Read the model definition and answer for the solid it produces. Units are mm, in the model's axes. A direction names the side the tool comes from. Round coordinates to 2 decimals unless told otherwise and drop trailing zeros. Write each loop counter-clockwise with the first axis right and the second up, starting at its lowest first coordinate (ties: lowest second). Pieces come first, ordered by that corner, then holes.
from build123d import *

# Parameters (mm, degrees)
SKETCH3_R           = 18.499963
BOSS_EXTRUDE1_DEPTH = 57.8000114
SKETCH4_R           = 2.999994
BOSS_EXTRUDE2_DEPTH = 20.00001334
SKETCH6_R           = 6.0000007
BOSS_EXTRUDE3_DEPTH = 5.0000154
SKETCH8_R           = 1.25000004
CUT_EXTRUDE3_DEPTH  = 8.89
SKETCH7_W           = 3.305573972
SKETCH7_H           = 0.499999
CUT_EXTRUDE4_DEPTH  = 13.9999974


with BuildPart() as part:
    # Sketch3 → Boss-Extrude1 (new body)
    with BuildSketch(Plane.XY):
        Circle(SKETCH3_R)
    extrude(amount=-BOSS_EXTRUDE1_DEPTH)

    # Sketch4 → Boss-Extrude2 (add)
    with BuildSketch(Plane.XY):
        Circle(SKETCH4_R)
    extrude(amount=BOSS_EXTRUDE2_DEPTH)

    # Sketch6 → Boss-Extrude3 (add)
    with BuildSketch(Plane.XY):
        with Locations(Location((0, 0, 0), (0, 0, 180))):
            Circle(SKETCH6_R)
    extrude(amount=BOSS_EXTRUDE3_DEPTH)

    # Sketch8 → Cut-Extrude3 (cut)
    with BuildSketch(Plane.XY):
        with Locations((0, 15.499969)):
            Circle(SKETCH8_R)
        with Locations((13.423366912, 7.7499845)):
            Circle(SKETCH8_R)
        with Locations((13.423366912, -7.7499845)):
            Circle(SKETCH8_R)
        with Locations((0, -15.499969)):
            Circle(SKETCH8_R)
        with Locations((-13.423366912, -7.7499845)):
            Circle(SKETCH8_R)
        with Locations((-13.423366912, 7.7499845)):
            Circle(SKETCH8_R)
    extrude(amount=-CUT_EXTRUDE3_DEPTH, mode=Mode.SUBTRACT)

    # Sketch7 → Cut-Extrude4 (cut)
    with BuildSketch(Plane.XY.offset(20.00001334)):
        with Locations((0, 2.753648673)):
            Rectangle(SKETCH7_W, SKETCH7_H)
    extrude(amount=-CUT_EXTRUDE4_DEPTH, mode=Mode.SUBTRACT)


solid = part.part
Q1. Flat-ended cylindrical pins translate along their axes: pin 1 Ø10 at (y, z) = (-12.5, -33.5) entering from +X; pin 2 Ø3 at (x, y) = (-14, 8) entering from +Z; pin 3 Ø3.5 at (x, y) = (2, 3) entering from +Z; pin 4 Ø2 at (x, z) = (-10.5, -2) entering from +Y. Find the tip coordinate at first contact, or state that the pin passes through.
Verdict:
pin 1: stops at x = 16.91
pin 2: stops at z = 0
pin 3: stops at z = 20
pin 4: stops at y = 15.87
Q2. Section A-A (x = 0) is taken. Determine the outline of the cut face in (y, z).
Verdict:
outline: (-18.5, -57.8) - (18.5, -57.8) - (18.5, 0) - (16.75, 0) - (16.75, -8.89) - (14.25, -8.89) - (14.25, 0) - (6, 0) - (6, 5) - (3, 5) - (3, 6) - (2.5, 6) - (2.5, 20) - (-3, 20) - (-3, 5) - (-6, 5) - (-6, 0) - (-14.25, 0) - (-14.25, -8.89) - (-16.75, -8.89) - (-16.75, 0) - (-18.5, 0) - close
Q3. Section D-D (z = -16.5) is taken. Determine the outline of the cut face in (x, y).
Verdict:
outline: circle Ø37 at (0, 0)
Q4. Which of the six approach directions +Z, -Z, +X, -X, +Y, -Y give full straight-line access (tool end or side, diameter ignored) to faces 1 (the flat face through (-13, -8, -8.89)), 2 (the flat face through (0, 0, -57.8))?
Verdict:
face 1: +Z
face 2: -Z, +X, -X, +Y, -Y
Q5. Section B-B (y = 0) is taken. Determine the outline of the cut face in (x, z), then the cut area to 3 significant figures.
Verdict:
outline: (-18.5, -57.8) - (18.5, -57.8) - (18.5, 0) - (6, 0) - (6, 5) - (3, 5) - (3, 20) - (-3, 20) - (-3, 5) - (-6, 5) - (-6, 0) - (-18.5, 0) - close
area: 2,290 mm2
Q6. Determine the mould class of faces 3 (the flat face through (0, 2.504, 13)), 4 (the cylindrical face through (-0.65, -2.93, 12.4)), 5 (the cylindrical face through (-0.16, -14.26, -4.38)) for opening direction X: pulls with the +X half, pulls with the -X half, needs draft (parallel to the pull), parting line crosses it, or undercut.
Verdict:
face 3: needs draft
face 4: parting line crosses it
face 5: undercut
Q7. Section C-C (z = -8) is taken. Determine the outline of the cut face in (x, y).
Verdict:
outline: circle Ø37 at (0, 0); hole circle Ø2.5 at (-13.42, -7.75); hole circle Ø2.5 at (-13.42, 7.75); hole circle Ø2.5 at (0, -15.5); hole circle Ø2.5 at (0, 15.5); hole circle Ø2.5 at (13.42, -7.75); hole circle Ø2.5 at (13.42, 7.75)
Q8. Straight lines are drawn through the part: probe 1 along Y at (x, z) = (0, -4); probe 2 along Z at (x, y) = (9.5, -8.5); probe 3 along X at (y, z) = (8.5, -1). For each, find the intervals that lie inside material, in ascending order.
Verdict:
probe 1: y = -18.5 to -16.75, -14.25 to 14.25, 16.75 to 18.5
probe 2: z = -57.8 to 0
probe 3: x = -16.43 to -14.42, -12.42 to 12.42, 14.42 to 16.43
